from build123d import *

# Parameters (mm, degrees)
SKETCH1_W                 = 279.4
SKETCH1_H                 = 279.4
BASE_FLANGE1_DEPTH        = 0.75946
SKETCH4_R                 = 1
CUT_EXTRUDE1_DEPTH        = 396.131999184
EDGE_FLANGE1_DEPTH        = 277.4
EDGE_FLANGE1_BEND_DEPTH   = 277.4
EDGE_FLANGE1_BEND_2_DEPTH = 277.4
EDGE_FLANGE1_BEND_3_DEPTH = 277.4
CUT_EXTRUDE2_REACH        = 399.847
SKETCH17_R                = 6.35
SKETCH17_R_2              = 10.31875
SKETCH17_W                = 98
SKETCH17_H                = 40
SKETCH19_R                = 1.75
CUT_EXTRUDE4_DEPTH        = 398.847258327


# Sheet-metal steps are written as plain solids
with BuildPart() as part:
    # Sketch1 → Base-Flange1 (new body)
    with BuildSketch(Plane(origin=(0, 0, 0), x_dir=(1, 0, 0), z_dir=(0, 1, 0))):
        with Locations((139.7, 139.7)):
            Rectangle(SKETCH1_W, SKETCH1_H)
    extrude(amount=BASE_FLANGE1_DEPTH)

    # Sketch4 → Cut-Extrude1 (cut, through all)
    with BuildSketch(Plane(origin=(0, 0.75946, 0), x_dir=(1, 0, 0), z_dir=(0, 1, 0))):
        Circle(SKETCH4_R)
        with Locations((0, 279.4)):
            Circle(SKETCH4_R)
        with Locations((279.4, 279.4)):
            Circle(SKETCH4_R)
        with Locations((279.4, 0)):
            Circle(SKETCH4_R)
    extrude(amount=-CUT_EXTRUDE1_DEPTH, mode=Mode.SUBTRACT)

    # Edge-Flange1 section (across the edge) → Edge-Flange1 (add)
    with BuildSketch(Plane(origin=(278.4, 0.75946, -280.4), x_dir=(0, 0, 1), z_dir=(-1, 0, 0))):
        with BuildLine():
            Line((-0.75946, 1), (-0.75946, 12.7))
            Line((-0.75946, 12.7), (0, 12.7))
            Line((0, 12.7), (0, 1))
            ThreePointArc((0, 1), (0.292893219, 0.292893219), (1, 0))
            Line((1, 0), (1, -0.75946))
            ThreePointArc((1, -0.75946), (-0.244126097, -0.244126097), (-0.75946, 1))
        make_face()
    extrude(amount=EDGE_FLANGE1_DEPTH)

    # Edge-Flange1 section 2 (across the edge) → Edge-Flange1 bend (add)
    with BuildSketch(Plane(origin=(-1, 0.75946, -278.4), x_dir=(1, 0, 0), z_dir=(0, 0, 1))):
        with BuildLine():
            Line((-0.75946, 1), (-0.75946, 12.7))
            Line((-0.75946, 12.7), (0, 12.7))
            Line((0, 12.7), (0, 1))
            ThreePointArc((0, 1), (0.292893219, 0.292893219), (1, 0))
            Line((1, 0), (1, -0.75946))
            ThreePointArc((1, -0.75946), (-0.244126097, -0.244126097), (-0.75946, 1))
        make_face()
    extrude(amount=EDGE_FLANGE1_BEND_DEPTH)

    # Edge-Flange1 section 3 (across the edge) → Edge-Flange1 bend 2 (add)
    with BuildSketch(Plane(origin=(1, 0.75946, 1), x_dir=(0, 0, -1), z_dir=(1, 0, 0))):
        with BuildLine():
            Line((-0.75946, 1), (-0.75946, 12.7))
            Line((-0.75946, 12.7), (0, 12.7))
            Line((0, 12.7), (0, 1))
            ThreePointArc((0, 1), (0.292893219, 0.292893219), (1, 0))
            Line((1, 0), (1, -0.75946))
            ThreePointArc((1, -0.75946), (-0.244126097, -0.244126097), (-0.75946, 1))
        make_face()
    extrude(amount=EDGE_FLANGE1_BEND_2_DEPTH)

    # Edge-Flange1 section 4 (across the edge) → Edge-Flange1 bend 3 (add)
    with BuildSketch(Plane(origin=(280.4, 0.75946, -1), x_dir=(-1, 0, 0), z_dir=(0, 0, -1))):
        with BuildLine():
            Line((-0.75946, 1), (-0.75946, 12.7))
            Line((-0.75946, 12.7), (0, 12.7))
            Line((0, 12.7), (0, 1))
            ThreePointArc((0, 1), (0.292893219, 0.292893219), (1, 0))
            Line((1, 0), (1, -0.75946))
            ThreePointArc((1, -0.75946), (-0.244126097, -0.244126097), (-0.75946, 1))
        make_face()
    extrude(amount=EDGE_FLANGE1_BEND_3_DEPTH)

    # Sketch17 → Cut-Extrude2 (cut, up to next)
    with BuildSketch(Plane.XZ, mode=Mode.PRIVATE) as cut_extrude2_sk1:
        with Locations(Location((25, -254.4, 0), (0, 0, 270))):
            Circle(SKETCH17_R)
    cut_extrude2_tool1 = extrude(cut_extrude2_sk1.sketch, amount=-CUT_EXTRUDE2_REACH, mode=Mode.PRIVATE) & part.part
    # Sketch17 → Cut-Extrude2 (cut, up to next)
    with BuildSketch(Plane.XZ, mode=Mode.PRIVATE) as cut_extrude2_sk2:
        with Locations(Location((63.1, -254.4, 0), (0, 0, 270))):
            Circle(SKETCH17_R_2)
    cut_extrude2_tool2 = extrude(cut_extrude2_sk2.sketch, amount=-CUT_EXTRUDE2_REACH, mode=Mode.PRIVATE) & part.part
    # Sketch17 → Cut-Extrude2 (cut, up to next)
    with BuildSketch(Plane.XZ, mode=Mode.PRIVATE) as cut_extrude2_sk3:
        with Locations(Location((227.84, -196.11, 0), (0, 0, 270))):
            Circle(SKETCH17_R_2)
    cut_extrude2_tool3 = extrude(cut_extrude2_sk3.sketch, amount=-CUT_EXTRUDE2_REACH, mode=Mode.PRIVATE) & part.part
    # Sketch17 → Cut-Extrude2 (cut, up to next)
    with BuildSketch(Plane.XZ, mode=Mode.PRIVATE) as cut_extrude2_sk4:
        with Locations((139.7, -75)):
            Rectangle(SKETCH17_W, SKETCH17_H)
    cut_extrude2_tool4 = extrude(cut_extrude2_sk4.sketch, amount=-CUT_EXTRUDE2_REACH, mode=Mode.PRIVATE) & part.part
    # Sketch17 → Cut-Extrude2 (cut, up to next)
    with BuildSketch(Plane.XZ, mode=Mode.PRIVATE) as cut_extrude2_sk5:
        with BuildLine():
            Line((128.7, -203), (150.7, -203))
            ThreePointArc((150.7, -203), (152.7, -205), (150.7, -207))
            Line((150.7, -207), (128.7, -207))
            ThreePointArc((128.7, -207), (126.7, -205), (128.7, -203))
        make_face()
    cut_extrude2_tool5 = extrude(cut_extrude2_sk5.sketch, amount=-CUT_EXTRUDE2_REACH, mode=Mode.PRIVATE) & part.part
    add(cut_extrude2_tool1.solids().sort_by_distance((25, 0, -254.4))[0], mode=Mode.SUBTRACT)
    add(cut_extrude2_tool2.solids().sort_by_distance((63.1, 0, -254.4))[0], mode=Mode.SUBTRACT)
    add(cut_extrude2_tool3.solids().sort_by_distance((227.84, 0, -196.11))[0], mode=Mode.SUBTRACT)
    add(cut_extrude2_tool4.solids().sort_by_distance((139.7, 0, -75))[0], mode=Mode.SUBTRACT)
    add(cut_extrude2_tool5.solids().sort_by_distance((139.7, 0, -205))[0], mode=Mode.SUBTRACT)

    # Sketch19 → Cut-Extrude4 (cut, through all)
    with BuildSketch(Plane.XZ):
        with Locations(Location((93.2, -47.5, 0), (0, 0, 270))):
            Circle(SKETCH19_R)
        with Locations(Location((186.2, -47.5, 0), (0, 0, 270))):
            Circle(SKETCH19_R)
        with Locations(Location((186.2, -102.5, 0), (0, 0, 270))):
            Circle(SKETCH19_R)
        with Locations(Location((93.2, -102.5, 0), (0, 0, 270))):
            Circle(SKETCH19_R)
    extrude(amount=-CUT_EXTRUDE4_DEPTH, mode=Mode.SUBTRACT)


solid = part.part
The listing builds one solid part. Answer for the finished solid, in the listing's coordinates (mm). A direction names the side the tool comes from. Coordinates: 2 decimals unless noted, no trailing zeros. Loops run counter-clockwise (first coordinate to the right, second up) from the corner with the lowest first, then second, coordinate; pieces in that order, holes last.
1) Flat-ended cylindrical pins translate along their axes: pin 1 Ø16.5 at (x, z) = (227.84, -196.11) entering from +Y; pin 2 Ø0.9 at (y, z) = (4.5, -280) entering from -X; pin 3 Ø23.5 at (x, z) = (63.1, -254.4) entering from +Y; pin 4 Ø0.6 at (x, y) = (115.5, 0.5) entering from +Z. Find the tip coordinate at first contact, or state that the pin passes through.
2) Find section A-A on z = -254.4. Write down the section's boundary in (x, y).
3) Find the intervals of material crossed by L1, parallel to Z at x = 93.2, y = 0.3; L2, parallel to X at y = 0.3, z = -102.5; L3, parallel to X at y = 9.5, z = -182, in increasing order.
4) Determine the mould class of faces 4 (the face through (138, 8, 1.759)), 5 (the face through (-1.759, 8, -142)), 6 (the face through (281.159, 8, -138)), 7 (the face through (280.4, 8, -138)) for opening direction X: pulls with the +X half, pulls with the -X half, needs draft (parallel to the pull), parting line crosses it, or undercut.
5) Find section B-B on x = 63.1. Write down the section's boundary in (y, z), then the cut area to 3 significant figures.
6) Find section C-C on y = 9.75. Write down the section's boundary in (x, z).
7) A tool of negligible diameter and unlimited length cuts with its end or side. For faces 1 (the face through (-1, 8, -142)), 2 (the face through (142, 8, -280.4)), 3 (the face through (138, 0.759, -142)), from which of +Z, -Z, +X, -X, +Y, -Y can it reach the whole face along a straight path? Write none if from no direction.
8) Find section D-D on z = -196.11. Write down the section's boundary in (x, y), then the cut area to 3 significant figures.
Values:
1. pin 1: passes through
1. pin 2: stops at x = 1
1. pin 3: stops at y = 0.76
1. pin 4: stops at z = 1.47
2. outline: (-1.76, 1.76) arc R1.76 ccw to (0, 0) - (18.65, 0) - (18.65, 0.76) - (0, 0.76) arc R1 cw to (-1, 1.76) - (-1, 13.46) - (-1.76, 13.46) - close; (31.35, 0) - (52.78, 0) - (52.78, 0.76) - (31.35, 0.76) - close; (73.42, 0) - (279.4, 0) arc R1.76 ccw to (281.16, 1.76) - (281.16, 13.46) - (280.4, 13.46) - (280.4, 1.76) arc R1 cw to (279.4, 0.76) - (73.42, 0.76) - close
3. L1: z = -280.38 to -104.25, -100.75 to -95, -55 to -49.25, -45.75 to 0.98
3. L2: x = -0.98 to 91.45, 94.95 to 184.45, 187.95 to 280.38
3. L3: x = -1.76 to -1, 280.4 to 281.16
4. face 4: needs draft
4. face 5: pulls with the -X half
4. face 6: pulls with the +X half
4. face 7: undercut
5. outline: (0, -279.4) arc R1.76 ccw to (1.76, -281.16) - (13.46, -281.16) - (13.46, -280.4) - (1.76, -280.4) arc R1 cw to (0.76, -279.4) - (0.76, -264.72) - (0, -264.72) - close; (0, -244.08) - (0.76, -244.08) - (0.76, 0) arc R1 cw to (1.76, 1) - (13.46, 1) - (13.46, 1.76) - (1.76, 1.76) arc R1.76 ccw to (0, 0) - close
5. area: 218 mm2
6. outline: (-1.76, -278.4) - (-1, -278.4) - (-1, -1) - (-1.76, -1) - close; (1, -281.16) - (278.4, -281.16) - (278.4, -280.4) - (1, -280.4) - close; (1, 1) - (278.4, 1) - (278.4, 1.76) - (1, 1.76) - close; (280.4, -278.4) - (281.16, -278.4) - (281.16, -1) - (280.4, -1) - close
7. face 1: +Z, -Z, +Y
7. face 2: +X, -X, +Y
7. face 3: +Y
8. outline: (-1.76, 1.76) arc R1.76 ccw to (0, 0) - (217.52, 0) - (217.52, 0.76) - (0, 0.76) arc R1 cw to (-1, 1.76) - (-1, 13.46) - (-1.76, 13.46) - close; (238.16, 0) - (279.4, 0) arc R1.76 ccw to (281.16, 1.76) - (281.16, 13.46) - (280.4, 13.46) - (280.4, 1.76) arc R1 cw to (279.4, 0.76) - (238.16, 0.76) - close
8. area: 218 mm2
